Verification items for the finished model (mm, model axes). Round coordinates to 2 decimals unless told otherwise and drop trailing zeros. Loops run counter-clockwise (first coordinate to the right, second up) from the corner with the lowest first, then second, coordinate; pieces in that order, holes last. Notation, with made-up numbers: (20.25, 10) -> (52.25, 10) arc R23 ccw to (52.25, 34) -> close; hole circle Ø9 at (72, -17). An arc over 180 degrees is marked (long way). Use a Markdown table: item, result. Add a question column.
```python
from build123d import *

# Parameters (mm, degrees)
BOSS_EXTRU_1_DEPTH                          = 3
FRAISAGE_POUR_VIS_T_TE_FRAIS_E_M31_AT_COUNT = 2
FRAISAGE_POUR_VIS_T_TE_FRAIS_E_M31_AT_PITCH = 92.5
FRAISAGE_POUR_VIS_T_TE_FRAIS_E_M31_2_COUNT  = 2
FRAISAGE_POUR_VIS_T_TE_FRAIS_E_M31_2_PITCH  = 185
FRAISAGE_POUR_VIS_T_TE_FRAIS_E_M32_AT_COUNT = 2
FRAISAGE_POUR_VIS_T_TE_FRAIS_E_M32_AT_PITCH = 185
FRAISAGE_POUR_VIS_T_TE_FRAIS_E_M32_2_COUNT  = 2
FRAISAGE_POUR_VIS_T_TE_FRAIS_E_M32_2_PITCH  = 92.5
FRAISAGE_POUR_VIS_T_TE_FRAIS_E_M33_AT_COUNT = 2
FRAISAGE_POUR_VIS_T_TE_FRAIS_E_M33_AT_PITCH = 226
FRAISAGE_POUR_VIS_T_TE_FRAIS_E_M33_2_COUNT  = 2
FRAISAGE_POUR_VIS_T_TE_FRAIS_E_M33_2_PITCH  = 222.583927109
FRAISAGE_POUR_VIS_T_TE_FRAIS_E_M33_3_COUNT  = 2
FRAISAGE_POUR_VIS_T_TE_FRAIS_E_M33_3_PITCH  = 235.236781008
FRAISAGE_POUR_VIS_T_TE_FRAIS_E_M33_4_COUNT  = 2
FRAISAGE_POUR_VIS_T_TE_FRAIS_E_M33_4_PITCH  = 116.302807958
FRAISAGE_POUR_VIS_T_TE_FRAIS_E_M33_5_COUNT  = 2
FRAISAGE_POUR_VIS_T_TE_FRAIS_E_M33_5_PITCH  = 87.940915433
FRAISAGE_POUR_VIS_T_TE_FRAIS_E_M33_6_COUNT  = 2
FRAISAGE_POUR_VIS_T_TE_FRAIS_E_M33_6_PITCH  = 28.963692658
FRAISAGE_POUR_VIS_T_TE_FRAIS_E_M33_7_COUNT  = 2
FRAISAGE_POUR_VIS_T_TE_FRAIS_E_M33_7_PITCH  = 227.84840463
FRAISAGE_POUR_VIS_T_TE_FRAIS_E_M33_8_COUNT  = 2
FRAISAGE_POUR_VIS_T_TE_FRAIS_E_M33_8_PITCH  = 25.401771592
FRAISAGE_POUR_VIS_T_TE_FRAIS_E_M33_9_COUNT  = 2
FRAISAGE_POUR_VIS_T_TE_FRAIS_E_M33_9_PITCH  = 206.046718003
FRAISAGE_POUR_VIS_T_TE_FRAIS_E_M33_10_COUNT = 2
FRAISAGE_POUR_VIS_T_TE_FRAIS_E_M33_10_PITCH = 210.150080353
FRAISAGE_POUR_VIS_T_TE_FRAIS_E_M33_11_COUNT = 2
FRAISAGE_POUR_VIS_T_TE_FRAIS_E_M33_11_PITCH = 48.508311372


with BuildPart() as part:
    # Esquisse2 → Boss.-Extru.1 (new body)
    with BuildSketch(Plane.XY):
        Polygon((-21.981846329, 125), (-21.981846329, 100), (-175, 100), (-175, -100), (-21.981846329, -100), (-21.981846329, -125), (21.981846329, -125), (21.981846329, -100), (175, -100), (175, 100), (21.981846329, 100), (21.981846329, 125), align=None)
    extrude(amount=BOSS_EXTRU_1_DEPTH)

    # Esquisse7 → Fraisage pour vis à tête fraisée M31 (revolve, cut)
    with BuildSketch(Plane(origin=(167.5, 92.5, 0), x_dir=(0, 1, 0), z_dir=(1, 0, 0))):
        Polygon((0, 0), (0, 3), (1.7, 3), (1.7, 1.45), (3.15, 0), align=None)
    fraisage_pour_vis_t_te_frais_e_m31 = revolve(axis=Axis((167.5, 92.5, -6.35), (0, 0, 1)), mode=Mode.SUBTRACT)

    # Fraisage pour vis à tête fraisée M31 at: Fraisage pour vis à tête fraisée M31 ×2
    with Locations(*[(0, -i * FRAISAGE_POUR_VIS_T_TE_FRAIS_E_M31_AT_PITCH, 0) for i in range(1, FRAISAGE_POUR_VIS_T_TE_FRAIS_E_M31_AT_COUNT)]):
        add(fraisage_pour_vis_t_te_frais_e_m31, mode=Mode.SUBTRACT)

    # Fraisage pour vis _ t_te frais_e M31 2: Fraisage pour vis à tête fraisée M31 ×2
    with Locations(*[(0, -i * FRAISAGE_POUR_VIS_T_TE_FRAIS_E_M31_2_PITCH, 0) for i in range(1, FRAISAGE_POUR_VIS_T_TE_FRAIS_E_M31_2_COUNT)]):
        add(fraisage_pour_vis_t_te_frais_e_m31, mode=Mode.SUBTRACT)

    # Esquisse9 → Fraisage pour vis à tête fraisée M32 (revolve, cut)
    with BuildSketch(Plane(origin=(-167.5, 92.5, 0), x_dir=(0, 1, 0), z_dir=(1, 0, 0))):
        Polygon((0, 0), (0, 3), (1.7, 3), (1.7, 1.45), (3.15, 0), align=None)
    fraisage_pour_vis_t_te_frais_e_m32 = revolve(axis=Axis((-167.5, 92.5, -6.35), (0, 0, 1)), mode=Mode.SUBTRACT)

    # Fraisage pour vis à tête fraisée M32 at: Fraisage pour vis à tête fraisée M32 ×2
    with Locations(*[(0, -i * FRAISAGE_POUR_VIS_T_TE_FRAIS_E_M32_AT_PITCH, 0) for i in range(1, FRAISAGE_POUR_VIS_T_TE_FRAIS_E_M32_AT_COUNT)]):
        add(fraisage_pour_vis_t_te_frais_e_m32, mode=Mode.SUBTRACT)

    # Fraisage pour vis _ t_te frais_e M32 2: Fraisage pour vis à tête fraisée M32 ×2
    with Locations(*[(0, -i * FRAISAGE_POUR_VIS_T_TE_FRAIS_E_M32_2_PITCH, 0) for i in range(1, FRAISAGE_POUR_VIS_T_TE_FRAIS_E_M32_2_COUNT)]):
        add(fraisage_pour_vis_t_te_frais_e_m32, mode=Mode.SUBTRACT)

    # Esquisse10 → Fraisage pour vis à tête fraisée M33 (revolve, cut)
    with BuildSketch(Plane(origin=(14.481846329, -113, 0), x_dir=(0, 1, 0), z_dir=(1, 0, 0))):
        Polygon((0, 0), (0, 3), (1.7, 3), (1.7, 1.45), (3.15, 0), align=None)
    fraisage_pour_vis_t_te_frais_e_m33 = revolve(axis=Axis((14.481846329, -113, -6.35), (0, 0, 1)), mode=Mode.SUBTRACT)

    # Fraisage pour vis à tête fraisée M33 at: Fraisage pour vis à tête fraisée M33 ×2
    with Locations(*[(0, i * FRAISAGE_POUR_VIS_T_TE_FRAIS_E_M33_AT_PITCH, 0) for i in range(1, FRAISAGE_POUR_VIS_T_TE_FRAIS_E_M33_AT_COUNT)]):
        add(fraisage_pour_vis_t_te_frais_e_m33, mode=Mode.SUBTRACT)

    # Fraisage pour vis _ t_te frais_e M33 2: Fraisage pour vis à tête fraisée M33 ×2
    with Locations(*[Vector(0.3842063296372473, 0.9232472563006483, 0) * (i * FRAISAGE_POUR_VIS_T_TE_FRAIS_E_M33_2_PITCH) for i in range(1, FRAISAGE_POUR_VIS_T_TE_FRAIS_E_M33_2_COUNT)]):
        add(fraisage_pour_vis_t_te_frais_e_m33, mode=Mode.SUBTRACT)

    # Fraisage pour vis _ t_te frais_e M33 3: Fraisage pour vis à tête fraisée M33 ×2
    with Locations(*[Vector(-0.4866664381255049, 0.8735878765197204, 0) * (i * FRAISAGE_POUR_VIS_T_TE_FRAIS_E_M33_3_PITCH) for i in range(1, FRAISAGE_POUR_VIS_T_TE_FRAIS_E_M33_3_COUNT)]):
        add(fraisage_pour_vis_t_te_frais_e_m33, mode=Mode.SUBTRACT)

    # Fraisage pour vis _ t_te frais_e M33 4: Fraisage pour vis à tête fraisée M33 ×2
    with Locations(*[Vector(-0.9843429263584751, 0.1762640159761305, 0) * (i * FRAISAGE_POUR_VIS_T_TE_FRAIS_E_M33_4_PITCH) for i in range(1, FRAISAGE_POUR_VIS_T_TE_FRAIS_E_M33_4_COUNT)]):
        add(fraisage_pour_vis_t_te_frais_e_m33, mode=Mode.SUBTRACT)

    # Fraisage pour vis _ t_te frais_e M33 5: Fraisage pour vis à tête fraisée M33 ×2
    with Locations(*[Vector(0.9724501189162041, 0.23311105984028424, 0) * (i * FRAISAGE_POUR_VIS_T_TE_FRAIS_E_M33_5_PITCH) for i in range(1, FRAISAGE_POUR_VIS_T_TE_FRAIS_E_M33_5_COUNT)]):
        add(fraisage_pour_vis_t_te_frais_e_m33, mode=Mode.SUBTRACT)

    # Fraisage pour vis _ t_te frais_e M33 6: Fraisage pour vis à tête fraisée M33 ×2
    with Locations(*[(-i * FRAISAGE_POUR_VIS_T_TE_FRAIS_E_M33_6_PITCH, 0, 0) for i in range(1, FRAISAGE_POUR_VIS_T_TE_FRAIS_E_M33_6_COUNT)]):
        add(fraisage_pour_vis_t_te_frais_e_m33, mode=Mode.SUBTRACT)

    # Fraisage pour vis _ t_te frais_e M33 7: Fraisage pour vis à tête fraisée M33 ×2
    with Locations(*[Vector(-0.12711825964048365, 0.9918875682586079, 0) * (i * FRAISAGE_POUR_VIS_T_TE_FRAIS_E_M33_7_PITCH) for i in range(1, FRAISAGE_POUR_VIS_T_TE_FRAIS_E_M33_7_COUNT)]):
        add(fraisage_pour_vis_t_te_frais_e_m33, mode=Mode.SUBTRACT)

    # Fraisage pour vis _ t_te frais_e M33 8: Fraisage pour vis à tête fraisée M33 ×2
    with Locations(*[Vector(0.5905099943842171, 0.8070303256584302, 0) * (i * FRAISAGE_POUR_VIS_T_TE_FRAIS_E_M33_8_PITCH) for i in range(1, FRAISAGE_POUR_VIS_T_TE_FRAIS_E_M33_8_COUNT)]):
        add(fraisage_pour_vis_t_te_frais_e_m33, mode=Mode.SUBTRACT)

    # Fraisage pour vis _ t_te frais_e M33 9: Fraisage pour vis à tête fraisée M33 ×2
    with Locations(*[Vector(0.07279902415018125, 0.9973466308574875, 0) * (i * FRAISAGE_POUR_VIS_T_TE_FRAIS_E_M33_9_PITCH) for i in range(1, FRAISAGE_POUR_VIS_T_TE_FRAIS_E_M33_9_COUNT)]):
        add(fraisage_pour_vis_t_te_frais_e_m33, mode=Mode.SUBTRACT)

    # Fraisage pour vis _ t_te frais_e M33 10: Fraisage pour vis à tête fraisée M33 ×2
    with Locations(*[Vector(-0.20920140779710872, 0.9778725739970969, 0) * (i * FRAISAGE_POUR_VIS_T_TE_FRAIS_E_M33_10_PITCH) for i in range(1, FRAISAGE_POUR_VIS_T_TE_FRAIS_E_M33_10_COUNT)]):
        add(fraisage_pour_vis_t_te_frais_e_m33, mode=Mode.SUBTRACT)

    # Fraisage pour vis _ t_te frais_e M33 11: Fraisage pour vis à tête fraisée M33 ×2
    with Locations(*[Vector(-0.90631257644203, 0.4226079906757676, 0) * (i * FRAISAGE_POUR_VIS_T_TE_FRAIS_E_M33_11_PITCH) for i in range(1, FRAISAGE_POUR_VIS_T_TE_FRAIS_E_M33_11_COUNT)]):
        add(fraisage_pour_vis_t_te_frais_e_m33, mode=Mode.SUBTRACT)


solid = part.part
```
1) Sectioned sample at B-B on x = 90. Enter the section's corners in (y, z), then the cut area to 3 significant figures.
2) Sectioned sample at C-C on y = -103.5. Enter the section's corners in (x, z).
3) Thickness scan on line 1 (Y direction, x = -167.5, z = 2.2); line 2 (X direction, y = 0, z = 2.4); line 3 (Y direction, x = 28.5, z = 0.25). Record the ranges inside material, lowest first.
4) Go/stop test with flat-tipped pins: pin 1 (2.5 mm diameter, centred on x = -167.5, y = -92.5, fed in from -Z); pin 2 (1.5 mm diameter, centred on y = 114, z = 1, fed in from -X); pin 3 (2 mm diameter, centred on x = -36, y = 15.5, fed in from -Z); pin 4 (1.5 mm diameter, centred on y = -110.5, z = 1, fed in from +X). Record where each tip stops, or that it passes through.
5) Sectioned sample at A-A on z = 0.75. State how many separate pieces and enclosed holes the cut face has, then the cut area to 3 significant figures.
Geometry results:
| question | item | result |
|---|---|---|
| 1 | outline | (-100, 0) -> (100, 0) -> (100, 3) -> (-100, 3) -> close |
| 1 | area | 600 mm^2 |
| 2 | outline | (-21.98, 0) -> (21.98, 0) -> (21.98, 3) -> (-21.98, 3) -> close |
| 3 | line 1 | -100 to -94.2, -90.8 to -1.7, 1.7 to 90.8, 94.2 to 100 |
| 3 | line 2 | -175 to -169.2, -165.8 to 165.8, 169.2 to 175 |
| 3 | line 3 | -100 to -95.23, -89.77 to 89.77, 95.23 to 100 |
| 4 | pin 1 | through |
| 4 | pin 2 | x = -21.98 |
| 4 | pin 3 | z = 0 |
| 4 | pin 4 | x = 21.98 |
| 5 | separate pieces | 1 |
| 5 | enclosed holes | 18 |
| 5 | area | 71,900 mm^2 |
